The listing builds one solid part. Answer for the finished solid, in the listing's coordinates (mm). A direction names the side the tool comes from. Coordinates: 2 decimals unless noted, no trailing zeros. Order: outer loops, then holes, each group sorted by start corner. A loop starts at its lowest first (then second) coordinate and runs counter-clockwise, first axis right, second up.
from build123d import *

# Parameters (mm, degrees)
BOSS_EXTRUDE1_DEPTH = 519.5
FILLET1_R           = 15
SKETCH2_W           = 33
SKETCH2_H           = 202
CUT_EXTRUDE1_DEPTH  = 54.5
FILLET2_R           = 10
CUT_EXTRUDE2_DEPTH  = 60.3400001


with BuildPart() as part:
    # Sketch1 → Boss-Extrude1 (new body, symmetric)
    with BuildSketch(Plane.XY):
        with BuildLine():
            Line((-40.754430434, 5), (-64.145425402, 5))
            ThreePointArc((-64.145425402, 5), (0, 64.34), (64.145425402, 5))
            Line((64.145425402, 5), (40.754430434, 5))
            ThreePointArc((40.754430434, 5), (0, 41.06), (-40.754430434, 5))
        make_face()
    extrude(amount=BOSS_EXTRUDE1_DEPTH, both=True)

    # Fillet1
    fillet1_edges = [part.edges().sort_by_distance(p)[0] for p in [
        (-52.449927918, 5, 519.5),
        (-52.449927918, 5, -519.5),
        (52.449927918, 5, -519.5),
        (52.449927918, 5, 519.5),
    ]]
    fillet(fillet1_edges, radius=FILLET1_R)

    # Sketch2 → Cut-Extrude1 (cut)
    with BuildSketch(Plane(origin=(0, 0, 0), x_dir=(1, 0, 0), z_dir=(0, 1, 0))):
        with Locations((0, -163)):
            Rectangle(SKETCH2_W, SKETCH2_H)
    extrude(amount=CUT_EXTRUDE1_DEPTH, mode=Mode.SUBTRACT)

    # Fillet2
    fillet2_edges = [part.edges().sort_by_distance(p)[0] for p in [
        (-16.5, 46.049425523, 62),
        (-16.5, 46.049425523, 264),
        (16.5, 46.049425523, 264),
        (16.5, 46.049425523, 62),
    ]]
    fillet(fillet2_edges, radius=FILLET2_R)

    # Sketch3 → Cut-Extrude2 (cut, through all)
    with BuildSketch(Plane.XZ.offset(-5)):
        with BuildLine():
            Line((-5.999925402, 246), (6.000074598, 246))
            ThreePointArc((6.000074598, 246), (13.07114241, 243.071067812), (16.000074598, 236))
            Line((16.000074598, 236), (16.000074598, 207))
            ThreePointArc((16.000074598, 207), (13.07114241, 199.928932188), (6.000074598, 197))
            Line((6.000074598, 197), (-5.999925402, 197))
            ThreePointArc((-5.999925402, 197), (-13.070993214, 199.928932188), (-15.999925402, 207))
            Line((-15.999925402, 207), (-15.999925402, 236))
            ThreePointArc((-15.999925402, 236), (-13.070993214, 243.071067812), (-5.999925402, 246))
        make_face()
    extrude(amount=-CUT_EXTRUDE2_DEPTH, mode=Mode.SUBTRACT)


solid = part.part
1) Consider L1, parallel to Z at x = -10, y = 61.5; L2, parallel to X at y = 37, z = -264; L3, parallel to X at y = 10.5, z = -437. Determine where each line is inside the solid, lowest interval first.
2) Each of these flat-tipped pins is pushed along its axis until it touches: P1, Ø5, axis at y = 45, z = 117.5, coming from the -X side; P2, Ø12, axis at y = 55, z = -164.5, coming from the +X side; P3, Ø18.5, axis at y = 44.5, z = 176, coming from the -X side; P4, Ø10, axis at x = -8, z = 209.5, coming from the -Y side. Where does it stop, or does it pass through?
3) Determine the mould class of faces 3 (the face through (1, 42, 519.5)), 4 (the face through (1, 42, -519.5)), 5 (the face through (-1.345, 64.326, 7.273)), 6 (the face through (-16.5, 46, 164)) for opening direction Z: released by +Z, released by -Z, zero draft, split by the parting line, or undercut.
4) Section A-A (z = 149.5) is taken. Give the vertices of the cut face in (x, y).
5) Section C-C (z = -162.5) is taken. Give the vertices of the cut face in (x, y).
6) A tool of negligible diameter and unlimited length cuts with its end or side. For faces 1 (the face through (53, 5, 7)), 2 (the face through (0, 54.5, 139)), from which of +Z, -Z, +X, -X, +Y, -Y can it reach the whole face along a straight path? Write none if from no direction.
7) Section B-B (x = 51) is taken. Give the vertices of the cut face in (y, z), then the cut area to 3 significant figures.
Filled sheet:
1. L1: z = -519.5 to 197.83, 245.17 to 519.5
1. L2: x = -52.64 to -17.8, 17.8 to 52.64
1. L3: x = -63.48 to -39.69, 39.69 to 63.48
2. P1: stops at x = -48.31
2. P2: stops at x = 41.7
2. P3: stops at x = -53.82
2. P4: passes through
3. face 3: released by +Z
3. face 4: released by -Z
3. face 5: zero draft
3. face 6: undercut
4. outline: (-64.15, 5) - (-40.75, 5) arc R41.06 cw to (-16.5, 37.6) - (-16.5, 54.5) - (16.5, 54.5) - (16.5, 37.6) arc R41.06 cw to (40.75, 5) - (64.15, 5) arc R64.34 ccw to start
5. outline: (-64.15, 5) - (-40.75, 5) arc R41.06 cw to (40.75, 5) - (64.15, 5) arc R64.34 ccw to start
6. face 1: +Z, -Z, +X, -X, -Y
6. face 2: -Y
7. outline: (5, -504.5) arc R15 ccw to (20, -519.5) - (39.23, -519.5) - (39.23, 519.5) - (20, 519.5) arc R15 ccw to (5, 504.5) - close
7. area: 35,500 mm2
